```python
from build123d import *

# Parameters (mm, degrees)
EXTRUDE_1_DEPTH          = 6
EXTRUDE_2_DEPTH          = 8
EXTRUDE_START            = -8
EXTRUDE_3_DEPTH          = 6
CUT_EXTRUDE_1_DEPTH      = 67.708320321
CUT_EXTRUDE_1_DEPTH_BACK = 8
SKETCH_3_R               = 2.75
FILLET_1_R               = 2
SKETCH_4_R               = 3.1
CUT_EXTRUDE_2_DEPTH      = 7


with BuildPart() as part:
    # 草图1 → 凸台-拉伸1 (new body)
    with BuildSketch(Plane(origin=(0, 0, 0), x_dir=(1, 0, 0), z_dir=(0, 1, 0))):
        Polygon((0, 0), (-45, 0), (0, 45), align=None)
    extrude(amount=EXTRUDE_1_DEPTH)

    # 草图2 → 凸台-拉伸2 (add)
    with BuildSketch(Plane.XZ):
        Polygon((-2.8, -42.2), (-2.8, -31.141125497), (-31.141125497, -2.8), (-42.2, -2.8), align=None)
    extrude(amount=EXTRUDE_2_DEPTH)

    # 草图1<3> → 凸台-拉伸3 (add)
    with BuildSketch(Plane(origin=(0, 0, 0), x_dir=(1, 0, 0), z_dir=(0, 1, 0)).offset(EXTRUDE_START)):
        Polygon((0, 0), (-45, 0), (0, 45), align=None)
    extrude(amount=-EXTRUDE_3_DEPTH)

    # 草图3 → 切除-拉伸1 (cut, two sides: drawn at the far end of the back side and taken through both)
    with BuildSketch(Plane.XZ.offset(14).offset(-CUT_EXTRUDE_1_DEPTH_BACK)):
        with Locations(Location((-13, -13, 0), (0, 0, 90))):
            Circle(SKETCH_3_R)
    extrude(amount=CUT_EXTRUDE_1_DEPTH + CUT_EXTRUDE_1_DEPTH_BACK, mode=Mode.SUBTRACT)

    # 圆角1
    # the kernel refuses this fillet: 2 mm, written as the material it takes off along each edge
    with BuildSketch(Plane(origin=(-2.8, 0, -31.141125497), x_dir=(0, 0, -1), z_dir=(0, -1, 0))) as fillet_1_piece_1:
        with BuildLine():
            CenterArc((FILLET_1_R * 0.414213562373, -FILLET_1_R), FILLET_1_R, 90, 45)
            Line((-FILLET_1_R * 0.292893218813, -FILLET_1_R * 0.292893218813), (0, 0))
            Line((0, 0), (FILLET_1_R * 0.414213562373, 0))
        make_face()
    extrude(amount=8, mode=Mode.SUBTRACT)
    with BuildSketch(Plane(origin=(-31.141125497, 0, -2.8), x_dir=(-1, 0, 0), z_dir=(0, -1, 0))) as fillet_1_piece_2:
        with BuildLine():
            CenterArc((FILLET_1_R * 0.414213562373, FILLET_1_R), FILLET_1_R, 225, 45)
            Line((-FILLET_1_R * 0.292893218813, FILLET_1_R * 0.292893218813), (0, 0))
            Line((0, 0), (FILLET_1_R * 0.414213562373, 0))
        make_face()
    extrude(amount=8, mode=Mode.SUBTRACT)
    with BuildSketch(Plane(origin=(-45, 4.071067812, 0), x_dir=(1, 0, 0), z_dir=(0, -1, 0)), Plane(origin=(-45, -12.071067812, 0), x_dir=(0.7071067811865471, 0, -0.7071067811865478), z_dir=(0, 1, 0))) as fillet_1_piece_3:
        with BuildLine():
            CenterArc((FILLET_1_R * 2.41421356237, -FILLET_1_R), FILLET_1_R, 90, 135)
            Line((FILLET_1_R * 1.70710678119, -FILLET_1_R * 1.70710678119), (0, 0))
            Line((0, 0), (FILLET_1_R * 2.41421356237, 0))
        make_face()
    extrude(amount=30.142135624, mode=Mode.SUBTRACT)
    with BuildSketch(Plane(origin=(0, 4.071067812, -45), x_dir=(0, 0, 1), z_dir=(0, -1, 0)), Plane(origin=(0, -12.071067812, -45), x_dir=(-0.7071067811865477, 0, 0.7071067811865474), z_dir=(0, 1, 0))) as fillet_1_piece_4:
        with BuildLine():
            CenterArc((FILLET_1_R * 2.41421356237, FILLET_1_R), FILLET_1_R, 135, 135)
            Line((FILLET_1_R * 1.70710678119, FILLET_1_R * 1.70710678119), (0, 0))
            Line((0, 0), (FILLET_1_R * 2.41421356237, 0))
        make_face()
    extrude(amount=30.142135624, mode=Mode.SUBTRACT)
    with BuildSketch(Plane(origin=(0, -3, 0), x_dir=(-1, 0, 0), z_dir=(0, -1, 0)), Plane(origin=(0, -5, 0), x_dir=(0, 0, -1), z_dir=(0, 1, 0))) as fillet_1_piece_5:
        with BuildLine():
            CenterArc((FILLET_1_R, FILLET_1_R), FILLET_1_R, 180, 90)
            Line((0, FILLET_1_R), (0, 0))
            Line((0, 0), (FILLET_1_R, 0))
        make_face()
    extrude(amount=16, mode=Mode.SUBTRACT)

    # 草图4 → 切除-拉伸2 (cut)
    with BuildSketch(Plane(origin=(0, 6, 0), x_dir=(1, 0, 0), z_dir=(0, 1, 0))):
        with Locations(Location((-11, 11, 0), (0, 0, 270))):
            Circle(SKETCH_4_R)
    extrude(amount=-CUT_EXTRUDE_2_DEPTH, mode=Mode.SUBTRACT)


solid = part.part
```
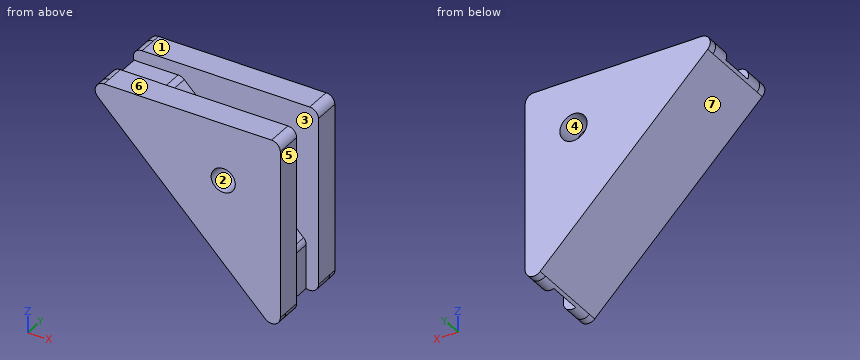
Geometry check sheet. Reference: the model listing, model coordinates, mm. Face numbers are marked on the shaded views. A direction names the side the tool comes from. Round coordinates to 2 decimals unless told otherwise and drop trailing zeros. Loops run counter-clockwise (first coordinate to the right, second up) from the corner with the lowest first, then second, coordinate; pieces in that order, holes last. Notation, with made-up numbers: (83, 78) - (122, 78) arc R21 ccw to (122, 93) - close; hole circle Ø2 at (18.25, 72). An arc over 180 degrees is marked (long way). Write item = value, one per line. Start each with the question number.
1. Section check D-D on z = -36.5. Enter the section's corners in (x, y).
2. Thickness scan on line 1 (Y direction, x = -19, z = -6.5); line 2 (X direction, y = 1.45, z = -11); line 3 (X direction, y = -11, z = -13). Record the ranges inside material, lowest first.
3. Depth check by flat-ended pin: pin 1 (3.5 mm diameter, centred on x = -11, z = -11, fed in from +Y); pin 2 (2 mm diameter, centred on x = -13.5, y = -3, fed in from +Z); pin 3 (8 mm diameter, centred on y = -6.5, z = -15, fed in from -X). Enter the tip coordinate at first touch or a pass-through.
4. Set-up check for the marked faces 1, 2 and 3: record each of +Z, -Z, +X, -X, +Y, -Y from which the full face is reachable in a straight line by a thin tool's end or side.
5. Section check B-B on x = -11. Enter the section's corners in (y, z), then the cut area to 3 significant figures.
6. Mould release check, pull along X, two halves, no side actions. Record for the marked faces 4, 5, 6 and 7: released by +X, released by -X, zero draft, split by the parting line, or undercut.
7. Section check A-A on y = 2.5. Enter the section's corners in (x, z), then the cut area to 3 significant figures.
8. Section check C-C on z = -11. Enter the section's corners in (x, y).
Working result:
q1.outline = (-8.5, -14) - (0, -14) - (0, -8) - (-2.8, -8) - (-2.8, 0) - (0, 0) - (0, 6) - (-8.5, 6) - close
q2.line_1 = -14 to -8, 0 to 6
q2.line_2 = -34 to -14.1, -7.9 to 0
q2.line_3 = -32 to -15.75, -10.25 to 0
q3.pin_1 = -8
q3.pin_2 = -19.44
q3.pin_3 = -34
q4.face_1 = +Z, +X, -X, +Y, -Y
q4.face_2 = -Y
q4.face_3 = +Z, +X
q5.outline = (-14, -34) - (6, -34) - (6, -14.1) - (0, -14.1) - (0, -22.94) - (-8, -22.94) - (-8, -14.89) - (-14, -14.89) - close; (-14, -11.11) - (-8, -11.11) - (-8, 0) - (-14, 0) - close; (0, -7.9) - (6, -7.9) - (6, 0) - (0, 0) - close
q5.area = 437 mm^2
q6.face_4 = undercut
q6.face_5 = released by +X
q6.face_6 = zero draft
q6.face_7 = released by -X
q7.outline = (-41.59, -3.41) - (-3.41, -41.59) arc R2 ccw to (0, -40.17) - (0, -2) arc R2 ccw to (-2, 0) - (-40.17, 0) arc R2 ccw to start; hole circle Ø6.2 at (-11, -11)
q7.area = 972 mm^2
q8.outline = (-34, -14) - (-14.89, -14) - (-14.89, -8) - (-22.94, -8) - (-22.94, 0) - (-14.1, 0) - (-14.1, 6) - (-34, 6) - close; (-11.11, -14) - (0, -14) - (0, -8) - (-11.11, -8) - close; (-7.9, 0) - (0, 0) - (0, 6) - (-7.9, 6) - close
